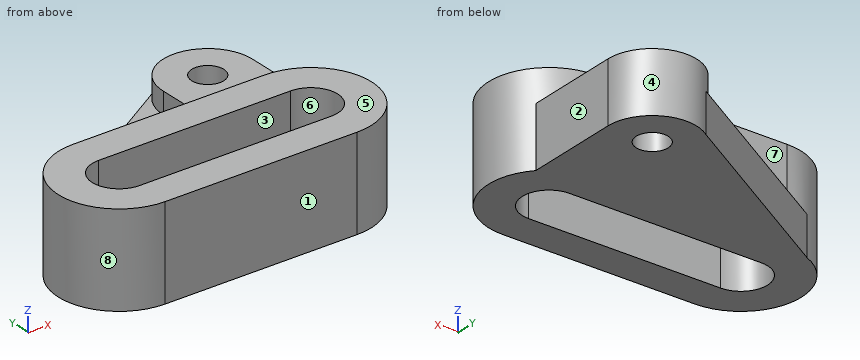
Autodesk Inventor part; units mm, degrees
ref_plane "Work Plane1" through (0, 0, 22) normal (0, 0, -1) x (-1, 0, 0)
ref_plane "YZ Plane" through (0, 0, 0) normal (1, 0, 0) x (0, 1, 0)
ref_plane "XZ Plane" through (0, 0, 0) normal (0, 1, 0) x (-1, 0, 0)
sketch "Sketch1" plane through (0, 0, 0) normal (0, 0, 1) x (1, 0, 0)
  line L0 (0, 0) -> (-108, 0) construction
  line L1 (0, -15) -> (-108, -15)
  line L2 (-108, 15) -> (0, 15)
  arc A0 (0, -15) -> (0, 15) centre (0, 0) ccw
  arc A1 (-108, 15) -> (-108, -15) centre (-108, 0) ccw
  line L3 (0, 0) -> (-108, 0) construction
  line L4 (0, -34) -> (-108, -34)
  line L5 (-108, 34) -> (0, 34)
  arc A2 (0, -34) -> (0, 34) centre (0, 0) ccw
  arc A3 (-108, 34) -> (-108, -34) centre (-108, 0) ccw
  point P0 (-54, 0)
  point P1 (-54, 0)
  dimension "d0" = 108
  dimension "d1" = 15
  dimension "d2" = 34
extrude "Extrusion1" add sketch "Sketch1" along normal blind 52
sketch "Sketch2" plane through (0, 0, 0) normal (0, 0, 1) x (1, 0, 0)
  arc A0 (-108, 15) -> (-108, -15) centre (-108, 0) ccw
  line L0 (-108, -15) -> (0, -15)
  arc A1 (0, -15) -> (0, 15) centre (0, 0) ccw
  line L1 (0, 15) -> (-108, 15)
  arc A2 (-108, 34) -> (-108, -34) centre (-108, 0) ccw
  line L2 (-108, 34) -> (0, 34)
  arc A3 (0, -34) -> (0, 34) centre (0, 0) ccw
  line L3 (0, -34) -> (-108, -34)
  circle A4 centre (0, 76) radius 9
  arc A5 (25, 76) -> (-25, 76) centre (0, 76) ccw
  line L4 (25, 76) -> (25, 23.0434)
  line L5 (-25, 76) -> (-25, 34)
  arc A6 (0, -34) -> (0, 34) centre (0, 0) ccw
  line L6 (-25, 34) -> (0, 34)
  arc A7 (-108, 15) -> (-108, -15) centre (-108, 0) ccw
  line L7 (-108, -15) -> (0, -15)
  arc A8 (0, -15) -> (0, 15) centre (0, 0) ccw
  line L8 (0, 15) -> (-108, 15)
  arc A9 (-108, 34) -> (-108, -34) centre (-108, 0) ccw
  line L9 (-108, 34) -> (0, 34)
  arc A10 (0, -34) -> (0, 34) centre (0, 0) ccw
  line L10 (0, -34) -> (-108, -34)
  arc A11 (-108, 15) -> (-108, -15) centre (-108, 0) ccw
  line L11 (-108, -15) -> (0, -15)
  arc A12 (0, -15) -> (0, 15) centre (0, 0) ccw
  line L12 (0, 15) -> (-108, 15)
  arc A13 (-108, 34) -> (-108, -34) centre (-108, 0) ccw
  line L13 (-108, 34) -> (0, 34)
  arc A14 (0, -34) -> (0, 34) centre (0, 0) ccw
  line L14 (0, -34) -> (-108, -34)
  arc A15 (25, 23.0434) -> (0, 34) centre (0, 0) ccw
  dimension "d5" = 18
  dimension "d6" = 76
  dimension "d7" = 61
  dimension "d8" = 25
  dimension "d9" = 34
extrude "Extrusion2" add sketch "Sketch2" along normal blind 34 contours L5 A5 L4 A3 L2
ref_plane "Work Plane1" through (0, 0, 22) normal (0, 0, -1) x (-1, 0, 0)
sketch "Sketch3" plane through (0, 0, 22) normal (0, 0, -1) x (-1, 0, 0)
  circle A0 centre (0, 76) radius 9
  arc A1 (108, -15) -> (108, 15) centre (108, 0) ccw
  line L0 (108, 15) -> (0, 15)
  arc A2 (0, 15) -> (0, -15) centre (0, 0) ccw
  line L1 (0, -15) -> (108, -15)
  arc A3 (108, -34) -> (108, 34) centre (108, 0) ccw
  line L2 (108, -34) -> (0, -34)
  arc A4 (-25, 23.0434) -> (0, -34) centre (0, 0) ccw
  line L3 (-25, 23.0434) -> (-25, 76)
  arc A5 (25, 76) -> (-25, 76) centre (0, 76) ccw
  line L4 (25, 76) -> (25, 34)
  line L5 (25, 34) -> (108, 34)
  arc A6 (25, 76) -> (-25, 76) centre (0, 76) ccw
  line L6 (14.6625, 96.2487) -> (121.2012, 31.3325)
  arc A7 (108, -34) -> (108, 34) centre (108, 0) ccw
extrude "Extrusion3" add sketch "Sketch3" along normal blind 22 contours A3 L5 L4 A5 L6
Geometry: final body of the model. Coordinates: model frame, mm. Face numbers are marked on the shaded views. A direction names the side the tool comes from. Give positions to 0.01 mm unless a question says otherwise; leave off trailing zeros. Loops run counter-clockwise (first coordinate to the right, second up) from the corner with the lowest first, then second, coordinate; pieces in that order, holes last. Notation, with made-up numbers: (6.25, 35) -> (62.25, 35) arc R30 ccw to (62.25, 65) -> close; hole circle Ø2 at (54.5, -5). An arc over 180 degrees is marked (long way). Use CSV: the item, a comma, the result in double quotes.
(1) Access query for the marked faces 1, 2, 3, 4 and 5. Directions: +Z, -Z, +X, -X, +Y, -Y. A direction counts if a zero-diameter tool reaches every point of the face in a straight line with its end or side. Return the directions, or none.
From the geometry:
face 1,"+Z, -Z, +X, -X, -Y"
face 2,"+Z, -Z, +X, +Y"
face 3,"+Z, -Z"
face 4,"+Z, +Y"
face 5,"+Z, +X, -X, +Y, -Y"
(2) Cut plane A-A (y = 0). Output: boundary loops of the cut face in (x, z), plus the area to 3 significant figures.
From the geometry:
outline,"(-142, 0) -> (-123, 0) -> (-123, 52) -> (-142, 52) -> close; (15, 0) -> (34, 0) -> (34, 52) -> (15, 52) -> close"
area,"1,980 mm^2"
(3) Cut plane B-B (x = -53.5). Output: boundary loops of the cut face in (y, z), plus the area to 3 significant figures.
From the geometry:
outline,"(-34, 0) -> (-15, 0) -> (-15, 52) -> (-34, 52) -> close; (15, 0) -> (72.58, 0) -> (72.58, 22) -> (34, 22) -> (34, 52) -> (15, 52) -> close"
area,"2,820 mm^2"
(4) Pull-direction query (X, two-part tool) for the marked faces 6, 7 and 8; classes: released by +X, released by -X, zero draft, split by the parting line, or undercut.
From the geometry:
face 6,"undercut"
face 7,"zero draft"
face 8,"released by -X"
(5) Ray query, line 1 along Y through (x, z) = (0, 9.5); line 2 along Y through (x, z) = (-99, 48.5); line 3 along Z through (x, y) = (-29.5, 38). Return the intervals inside material, ascending. Write a range as [from, to].
From the geometry:
line 1,"[-34, -15], [15, 67], [85, 101]"
line 2,"[-34, -15], [15, 34]"
line 3,"[0, 22]"
(6) Cut plane D-D (y = 41). Output: boundary loops of the cut face in (x, z).
From the geometry:
outline,"(-105.34, 0) -> (25, 0) -> (25, 34) -> (-25, 34) -> (-25, 22) -> (-105.34, 22) -> close"
(7) Cut plane C-C (z = 14.5). Output: boundary loops of the cut face in (x, y), plus the area to 3 significant figures.
From the geometry:
outline,"(-121.2, 31.33) arc R34 ccw to (-108, -34) -> (0, -34) arc R34 ccw to (25, 23.04) -> (25, 76) arc R25 ccw to (-14.66, 96.25) -> close; hole (-108, -15) -> (0, -15) arc R15 ccw to (0, 15) -> (-108, 15) arc R15 ccw to start; hole circle Ø18 at (0, 76)"
area,"12,500 mm^2"
(8) First-contact query: P1, Ø10, axis at x = -40.5, z = 22.5, coming from the +Y side; P2, Ø9, axis at x = -30, z = 42.5, coming from the +Y side; P3, Ø17, axis at y = 50, z = 11, coming from the +X side; P4, Ø12, axis at x = 4.5, z = 31, coming from the -Y side. Flat tips, straight axial feed; report the tip coordinate or a pass-through.
From the geometry:
P1,"y = 83.54"
P2,"y = 34"
P3,"x = 25"
P4,"y = -34"
